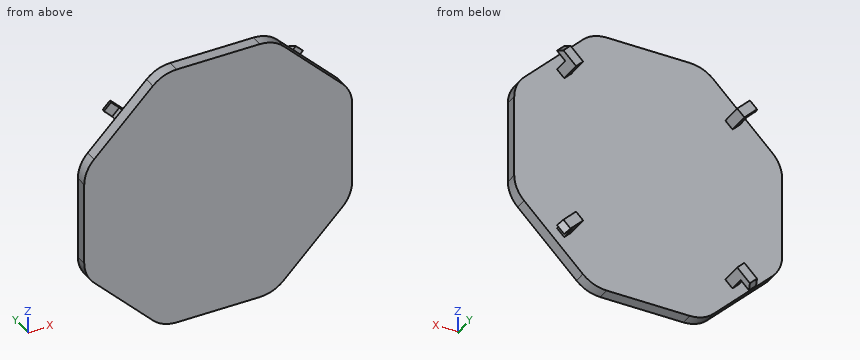
```python
from build123d import *

# Parameters (mm, degrees)
BOSS_EXTRUDE1_DEPTH = 3.5
FILLET1_R           = 10
BOSS_EXTRUDE2_DEPTH = 1.5
CIRPATTERN1_COUNT   = 4


with BuildPart() as part:
    # Sketch1 → Boss-Extrude1 (new body)
    with BuildSketch(Plane(origin=(0, 0, 0), x_dir=(1, 0, 0), z_dir=(0, 1, 0))):
        Polygon((40, 16.568542495), (16.568542495, 40), (-16.568542495, 40), (-40, 16.568542495), (-40, -16.568542495), (-16.568542495, -40), (16.568542495, -40), (40, -16.568542495), align=None)
    extrude(amount=BOSS_EXTRUDE1_DEPTH)

    # Fillet1
    fillet1_edges = [part.edges().sort_by_distance(p)[0] for p in [
        (40, 1.75, 16.568542495),
        (16.568542495, 1.75, 40),
        (-16.568542495, 1.75, 40),
        (-40, 1.75, 16.568542495),
        (-40, 1.75, -16.568542495),
        (-16.568542495, 1.75, -40),
        (16.568542495, 1.75, -40),
        (40, 1.75, -16.568542495),
    ]]
    fillet(fillet1_edges, radius=FILLET1_R)

    # Sketch3 → Boss-Extrude2 (add, symmetric)
    with BuildSketch(Plane(origin=(0, 0, 0), x_dir=(-0.707106781, 0, 0.707106781), z_dir=(-0.707106781, 0, -0.707106781))):
        Polygon((-33.97, 3.5), (-33.97, 10), (-39.315299462, 10), (-40.47, 8), (-36.97, 8), (-36.97, 3.5), align=None)
    boss_extrude2 = extrude(amount=BOSS_EXTRUDE2_DEPTH, both=True)

    # CirPattern1: Boss-Extrude2 ×4 about axis
    cirpattern1_axis = Axis((-0.042786503, 0, 0.042786503), (0, 1, 0))
    for i in range(1, CIRPATTERN1_COUNT):
        add(boss_extrude2.rotate(cirpattern1_axis, i * 360 / CIRPATTERN1_COUNT))


solid = part.part
```
Geometry: final body of the model. Coordinates: model frame, mm. Coordinates: 2 decimals unless noted, no trailing zeros. Order: outer loops, then holes, each group sorted by start corner. A loop starts at its lowest first (then second) coordinate and runs counter-clockwise, first axis right, second up.
Item 1: Section query A-A (y = 4.75). Output: boundary loops of the cut face in (x, z), then the cut area to 3 significant figures.
Answer:
outline: (-27.29, -25.08) - (-25.17, -27.2) - (-23.05, -25.08) - (-25.17, -22.96) - close; (-27.29, 25.17) - (-25.17, 23.05) - (-23.05, 25.17) - (-25.17, 27.29) - close; (22.96, -25.08) - (25.08, -27.2) - (27.2, -25.08) - (25.08, -22.96) - close; (22.96, 25.17) - (25.08, 23.05) - (27.2, 25.17) - (25.08, 27.29) - close
area: 36.0 mm2
Item 2: Section query C-C (z = 9.5). Output: boundary loops of the cut face in (x, y).
Answer:
outline: (-40, 0) - (40, 0) - (40, 3.5) - (-40, 3.5) - close
Item 3: Contact query for a flat-ended pin moving along its axis: P1, Ø5, axis at x = -20, y = 4.5, coming from the -Z side. Output: stop coordinate, or through.
Answer:
P1: stops at z = -38.49
Item 4: Section query D-D (x = -10.5). Output: boundary loops of the cut face in (y, z), then the cut area to 3 significant figures.
Answer:
outline: (0, -40) - (3.5, -40) - (3.5, 40) - (0, 40) - close
area: 280 mm2
Item 5: Section query B-B (x = -24). Output: boundary loops of the cut face in (y, z), then the cut area to 3 significant figures.
Answer:
outline: (0, -32.57) - (3.5, -32.57) - (3.5, -26.04) - (10, -26.04) - (10, -24.13) - (3.5, -24.13) - (3.5, 24.21) - (10, 24.21) - (10, 26.12) - (3.5, 26.12) - (3.5, 32.57) - (0, 32.57) - close
area: 253 mm2
Item 6: Material intervals for line 1 along Y through (x, z) = (11, 20.5); line 2 along Z through (x, y) = (19.5, 1.5); line 3 along X through (y, z) = (7.5, 24), sorted ascending.
Answer:
line 1: y = 0 to 3.5
line 2: z = -37.07 to 37.07
line 3: x = -26.12 to -24.21, 24.13 to 26.04
